Design review of the part built by this model. Coordinates are the model's own, in mm. Coordinates: 2 decimals unless noted, no trailing zeros. Write each loop counter-clockwise with the first axis right and the second up, starting at its lowest first coordinate (ties: lowest second). Pieces come first, ordered by that corner, then holes.
```python
from build123d import *

# Parameters (mm, degrees)
SKETCH_R     = 12.5
PAD_DEPTH    = 5
FILLET_R     = 1
SKETCH001_R  = 2.5
POCKET_DEPTH = 5
CHAMFER_SIZE = 2


with BuildPart() as part:
    # Sketch (on XY_Plane of Origin) → Pad (new body)
    with BuildSketch(Plane.XY):
        Circle(SKETCH_R)
    extrude(amount=PAD_DEPTH)

    # Fillet
    fillet_edges = [part.edges().sort_by_distance(p)[0] for p in [
        (-12.5, 0, 5),
        (-12.5, 0, 0),
    ]]
    fillet(fillet_edges, radius=FILLET_R)

    # Sketch001 (on Face5 of Fillet) → Pocket (cut)
    with BuildSketch(Plane.XY.offset(5)):
        Circle(SKETCH001_R)
    extrude(amount=-POCKET_DEPTH, mode=Mode.SUBTRACT)

    # Chamfer
    chamfer_edges = [part.edges().sort_by_distance(p)[0] for p in [
        (-2.5, 0, 5),
    ]]
    chamfer(chamfer_edges, length=CHAMFER_SIZE)


solid = part.part
```
(1) Consider section C-C (z = 3.4). Give the boundary of the cut face in (x, y), plus the area to 3 significant figures.
(2) Wall thickness on line 1 (Y direction, x = 0, z = 1.75); line 2 (X direction, y = 1.25, z = 3.4); line 3 (Y direction, x = 10, z = 4.3): over which ranges is each line inside the solid? List them lowest first.
(3) Mouldability with a two-part tool opening along X and no side actions: class faces 1 (the flat face through (-3, 0, 0)), 2 (the cylindrical face through (-0.54, -2.44, 1.52)), 3 (the cylindrical face through (11.923, 3.755, 2.479)) as +X half, -X half, draft (parallel to the pull), parting line (faces both ways), or undercut.
(4) Insertion check: pin 1 Ø2 at (x, z) = (-5, 3.5) entering from -Y; pin 2 Ø3 at (y, z) = (-4, 2) entering from +X. Each pin has a flat end and moves straight along its axis. Give the tip position at first contact, or say it passes through.
(5) Consider section A-A (x = 0). Give the boundary of the cut face in (y, z).
(6) Consider section D-D (z = 1.8). Give the boundary of the cut face in (x, y).
Results:
1. outline: circle Ø25 at (0, 0); hole circle Ø5.8 at (0, 0)
1. area: 464 mm2
2. line 1: y = -12.5 to -2.5, 2.5 to 12.5
2. line 2: x = -12.44 to -2.62, 2.62 to 12.44
2. line 3: y = -7.42 to 7.42
3. face 1: draft
3. face 2: undercut
3. face 3: parting line
4. pin 1: stops at y = -11.84
4. pin 2: stops at x = 12.25
5. outline: (-12.5, 1) arc R1 ccw to (-11.5, 0) - (-2.5, 0) - (-2.5, 3) - (-4.5, 5) - (-11.5, 5) arc R1 ccw to (-12.5, 4) - close; (2.5, 0) - (11.5, 0) arc R1 ccw to (12.5, 1) - (12.5, 4) arc R1 ccw to (11.5, 5) - (4.5, 5) - (2.5, 3) - close
6. outline: circle Ø25 at (0, 0); hole circle Ø5 at (0, 0)
